Source: CAD feature listing. Evaluate the final solid. Frame: model axes, mm. A direction names the side the tool comes from. Round coordinates to 2 decimals unless told otherwise and drop trailing zeros. Loops run counter-clockwise (first coordinate to the right, second up) from the corner with the lowest first, then second, coordinate; pieces in that order, holes last. Notation, with made-up numbers: (51, 51.5) -> (92, 51.5) arc R15 ccw to (92, 77.5) -> close; hole circle Ø6 at (78, -16.75). An arc over 180 degrees is marked (long way). Write item = value, one per line.
Autodesk Inventor part; units mm, degrees
ref_plane "YZ Plane" through (0, 0, 0) normal (1, 0, 0) x (0, 1, 0)
ref_plane "XZ Plane" through (0, 0, 0) normal (0, 1, 0) x (-1, 0, 0)
ref_plane "XY Plane" through (0, 0, 0) normal (0, 0, 1) x (1, 0, 0)
sketch "Boceto1" plane through (0, 0, 0) normal (0, 0, 1) x (1, 0, 0)
  circle A0 centre (0, 0) radius 4
  line L0 (0, 3.2332) -> (2.8, 1.6166)
  line L1 (2.8, 1.6166) -> (2.8, -1.6166)
  line L2 (2.8, -1.6166) -> (0, -3.2332)
  line L3 (0, -3.2332) -> (-2.8, -1.6166)
  line L4 (-2.8, -1.6166) -> (-2.8, 1.6166)
  line L5 (-2.8, 1.6166) -> (0, 3.2332)
  line L6 (0, -3.2332) -> (0, -4)
  point P0 (2.8, 0)
  dimension "d0" = 8
  dimension "d1" = 5.6
extrude "Extrusión1" add sketch "Boceto1" along normal blind 7
properties part number "AcopleRod"
1. Section query B-B (z = 3.5). Return the cut outline in (x, y), then the cut area to 3 significant figures.
Evaluation:
outline = circle Ø8 at (0, 0); hole (-2.8, -1.62) -> (0, -3.23) -> (2.8, -1.62) -> (2.8, 1.62) -> (0, 3.23) -> (-2.8, 1.62) -> close
area = 23.1 mm²
2. Line query: probe 1 along X at (y, z) = (0, 3.5); probe 2 along Y at (x, z) = (2.5, 3.75); probe 3 along X at (y, z) = (-2, 2.25). Output: solid intervals per line, ascending. Write a range as from..to.
Evaluation:
probe_1 = -4..-2.8, 2.8..4
probe_2 = -3.12..-1.79, 1.79..3.12
probe_3 = -3.46..-2.14, 2.14..3.46
3. Section query D-D (y = 3.75). Return the cut outline in (x, z).
Evaluation:
outline = (-1.39, 0) -> (1.39, 0) -> (1.39, 7) -> (-1.39, 7) -> close
4. Mould query, pull axis Y, two halves, no side actions, for faces 3 (the face through (-1, -3, 0)), 4 (the face through (-0.867, 3.905, 3.451)), 5 (the face through (-1.42, 2.414, 3.451)). Classes: released by +Y, released by -Y, zero draft, split by the parting line, or undercut.
Evaluation:
face_3 = zero draft
face_4 = split by the parting line
face_5 = undercut
5. Section query A-A (y = 0). Return the cut outline in (x, z), then the cut area to 3 significant figures.
Evaluation:
outline = (-4, 0) -> (-2.8, 0) -> (-2.8, 7) -> (-4, 7) -> close; (2.8, 0) -> (4, 0) -> (4, 7) -> (2.8, 7) -> close
area = 16.8 mm²
6. Set-up query: faces 1 (the face through (1.38, 2.436, 3.451)), 2 (the face through (-1, -3, 7)). Return all of +Z, -Z, +X, -X, +Y, -Y with unobstructed straight access to the full face (end or side cutting, diameter ignored); none if empty.
Evaluation:
face_1 = +Z, -Z
face_2 = +Z, +X, -X, +Y, -Y
7. Section query C-C (x = -2.25). Return the cut outline in (y, z).
Evaluation:
outline = (-3.31, 0) -> (-1.93, 0) -> (-1.93, 7) -> (-3.31, 7) -> close; (1.93, 0) -> (3.31, 0) -> (3.31, 7) -> (1.93, 7) -> close
